Autodesk Inventor part; units mm, degrees
ref_plane "YZ Plane" through (0, 0, 0) normal (1, 0, 0) x (0, 1, 0)
ref_plane "XZ Plane" through (0, 0, 0) normal (0, 1, 0) x (-1, 0, 0)
ref_plane "XY Plane" through (0, 0, 0) normal (0, 0, 1) x (1, 0, 0)
sketch "Sketch1" plane through (0, 0, 0) normal (0, 1, 0) x (-1, 0, 0)
  circle A0 centre (0, 0) radius 36
  dimension "d0" = 72
extrude "Extrusion1" add sketch "Sketch1" along normal blind 11
sketch "Sketch2" plane through (0, 0, 0) normal (0, -1, 0) x (1, 0, 0)
  line L0 (0, -58.3451) -> (0, 0) construction
  line L1 (0, 0) -> (-17.6777, -17.6777) construction
  point P0 (0, -25)
  point P1 (17.6777, -17.6777)
  point P2 (17.6777, 17.6777)
  point P3 (-17.6777, 17.6777)
  dimension "d84" = 45
  dimension "d85" = 25
  dimension "d86" = 25
  dimension "d89" = 360
fillet "Fillet2" radius 1 1 edges at (36, 0, 0)
sketch "Sketch10" plane through (0, 0, 0) normal (0, -1, 0) x (1, 0, 0)
  circle A0 centre (0, 0) radius 15
  dimension "d66" = 30
extrude "Extrusion6" add sketch "Sketch10" along normal blind 9
fillet "Fillet4" radius 3.175 1 edges at (-15, 0, 0)
sketch "Sketch11" plane through (0, -9, 0) normal (0, -1, 0) x (1, 0, 0)
  line L0 (-8.5, -4.2426) -> (-8.5, 4.2426)
  line L1 (8.5, 4.2426) -> (8.5, -4.2426)
  arc A0 (-8.5, -4.2426) -> (8.5, -4.2426) centre (0, 0) ccw
  arc A1 (8.5, 4.2426) -> (-8.5, 4.2426) centre (0, 0) ccw
  dimension "d71" = 17
  dimension "d72" = 8.5
  dimension "d73" = 9.5
  dimension "d74" = 9.5
extrude "Extrusion7" cut sketch "Sketch11" against normal blind 9
sketch "Sketch12" plane through (0, 11, 0) normal (0, 1, 0) x (1, 0, 0)
  point P0 (0, 0)
  point P1 (0, 0)
hole "Hole5" at (0, 11, 0) direction (0, -1, 0) diameter 6.2 end through all countersink diameter 13.44 countersink angle 90
hole "Hole6" at (-17.6777, 0, -17.6777) at (0, 0, -25) at (17.6777, 0, -17.6777) at (17.6777, 0, 17.6777) at (-17.6777, 0, 17.6777) direction (0, 1, 0) diameter 6.2 end through all
properties part number "baseplate" material "PBT Plastic"
Read the model definition and answer for the solid it produces. Units are mm, in the model's axes. A direction names the side the tool comes from. Give positions to 0.01 mm unless a question says otherwise; leave off trailing zeros. Order: outer loops, then holes, each group sorted by start corner. A loop starts at its lowest first (then second) coordinate and runs counter-clockwise, first axis right, second up. Notation, with made-up numbers: (88.5, 32.5) -> (111.5, 32.5) arc R15 ccw to (111.5, 57.5) -> close; hole circle Ø9 at (-38.5, 59). An arc over 180 degrees is marked (long way). One line per item, written item: value. Start each with the question number.
(1) Straight lines are drawn through the part: L1, parallel to Z at x = 0, y = 3.75; L2, parallel to Y at x = 19.5, z = 3; L3, parallel to X at y = 8, z = -22.5. For each, find the intervals that lie inside material, in ascending order.
(2) Flat-ended cylindrical pins translate along their axes: P1, Ø8, axis at x = -11.5, y = 3, coming from the -Z side; P2, Ø6, axis at x = 18.5, y = 7.5, coming from the -Z side; P3, Ø7, axis at y = -4.5, z = -0.5, coming from the -X side. Find the tip coordinate at first contact, or state that the pin passes through.
(3) The part is cut by section B-B (x = 0). Determine the outline of the cut face in (y, z) (3 decimals), and give its area (3 significant figures).
(4) The part is cut by section A-A (z = 0). Determine the outline of the cut face in (x, y) (3 decimals).
(5) For a pull along X with two mould halves and no side action, classify faces 3 (the flat face through (-4, 0, 0)), 4 (the flat face through (-15, 0, -15)), 5 (the cylindrical face through (-14.985, -6.047, -0.66)) as released by +X, released by -X, zero draft, split by the parting line, or undercut.
(6) The part is cut by section D-D (y = 8.25). Determine the outline of the cut face in (x, z), and give its area (3 significant figures).
(7) A tool of negligible diameter and unlimited length cuts with its end or side. For faces 1 (the cylindrical face through (0.1, -4.6, 9.5)), 2 (the cylindrical face through (-19.773, 5.577, 19.963)), from which of +Z, -Z, +X, -X, +Y, -Y can it reach the whole face along a straight path? Write none if from no direction.
(8) The part is cut by section C-C (y = -5.75). Determine the outline of the cut face in (x, z), and give its area (3 significant figures).
Taken from the geometry:
1. L1: -36 to -28.1, -21.9 to -3.1, 3.1 to 36
1. L2: 0 to 11
1. L3: -28.1 to -1.83, 1.83 to 28.1
2. P1: z = -35.21
2. P2: z = -32.49
2. P3: x = -15.86
3. outline: (-9, -15) -> (-3.175, -15) arc R3.175 cw to (0, -18.175) -> (0, -21.9) -> (11, -21.9) -> (11, -6.72) -> (7.38, -3.1) -> (0, -3.1) -> (0, -9.5) -> (-9, -9.5) -> close; (-9, 9.5) -> (0, 9.5) -> (0, 3.1) -> (7.38, 3.1) -> (11, 6.72) -> (11, 36) -> (1, 36) arc R1 ccw to (0, 35) -> (0, 18.175) arc R3.175 cw to (-3.175, 15) -> (-9, 15) -> close; (0, -35) arc R1 ccw to (1, -36) -> (11, -36) -> (11, -28.1) -> (0, -28.1) -> close
3. area: 745 mm^2
4. outline: (-36, 1) arc R1 ccw to (-35, 0) -> (-18.175, 0) arc R3.175 cw to (-15, -3.175) -> (-15, -9) -> (-8.5, -9) -> (-8.5, 0) -> (-3.1, 0) -> (-3.1, 7.38) -> (-6.72, 11) -> (-36, 11) -> close; (3.1, 0) -> (8.5, 0) -> (8.5, -9) -> (15, -9) -> (15, -3.175) arc R3.175 cw to (18.175, 0) -> (35, 0) arc R1 ccw to (36, 1) -> (36, 11) -> (6.72, 11) -> (3.1, 7.38) -> close
5. face 3: undercut
5. face 4: zero draft
5. face 5: split by the parting line
6. outline: circle Ø72 at (0, 0); hole circle Ø6.2 at (-17.68, -17.68); hole circle Ø6.2 at (-17.68, 17.68); hole circle Ø7.94 at (0, 0); hole circle Ø6.2 at (0, -25); hole circle Ø6.2 at (17.68, -17.68); hole circle Ø6.2 at (17.68, 17.68)
6. area: 3,870 mm^2
7. face 1: -Y
7. face 2: +Y, -Y
8. outline: circle Ø30 at (0, 0); hole (-8.5, -4.24) arc R9.5 ccw to (8.5, -4.24) -> (8.5, 4.24) arc R9.5 ccw to (-8.5, 4.24) -> close
8. area: 435 mm^2
